from build123d import *

# Parameters (mm, degrees)
SKETCH051_W         = 21.9
SKETCH051_H         = 24
PAD014_DEPTH        = 4
SKETCH052_R         = 5.9
POCKET015_DEPTH     = 1.2
SKETCH053_W         = 16
SKETCH053_H         = 6
SKETCH053_W_2       = 4
POCKET016_DEPTH     = 1.2
HOLE022_D           = 2.8
HOLE022_DEPTH       = 25
HOLE022_CBORE_D     = 6
HOLE022_CBORE_DEPTH = 2
FILLET027_R         = 2


with BuildPart() as part:
    # Sketch051 → Pad014 (new body)
    with BuildSketch(Plane.XY):
        with Locations((11.05, 0)):
            Rectangle(SKETCH051_W, SKETCH051_H)
    extrude(amount=PAD014_DEPTH)

    # Sketch052 (on Face6 of Pad014) → Pocket015 (cut)
    with BuildSketch(Plane.XY.offset(4)):
        with Locations((7.5, 0)):
            Circle(SKETCH052_R)
    pocket015 = extrude(amount=-POCKET015_DEPTH, mode=Mode.SUBTRACT)

    # Mirrored025: Pocket015 across Sketch052 V_Axis
    add(pocket015.mirror(Plane(origin=(0, 0, 4), x_dir=(0, 0, 1), z_dir=(1, 0, 0))), mode=Mode.SUBTRACT)

    # Sketch053 (on Face5 of Mirrored025) → Pocket016 (cut)
    with BuildSketch(Plane.XY.offset(4)):
        with Locations((0, 3)):
            Rectangle(SKETCH053_W, SKETCH053_H)
        with Locations((0, 9)):
            Rectangle(SKETCH053_W_2, SKETCH053_H)
    extrude(amount=-POCKET016_DEPTH, mode=Mode.SUBTRACT)

    # Hole022
    with Locations(Plane(origin=(0, 0, 0), x_dir=(1, 0, 0), z_dir=(0, 0, -1))):
        with Locations((16.2, 8.2), (16.2, -8.2), (3.8, 8.2), (3.8, -8.2)):
            hole022 = CounterBoreHole(HOLE022_D / 2, HOLE022_CBORE_D / 2, HOLE022_CBORE_DEPTH, depth=HOLE022_DEPTH)

    # Mirrored026: Hole022 across Sketch054 V_Axis
    add(hole022.mirror(Plane(origin=(0, 0, 0), x_dir=(0, 0, -1), z_dir=(1, 0, 0))), mode=Mode.SUBTRACT)

    # Fillet027
    fillet027_edges = [part.edges().sort_by_distance(p)[0] for p in [
        (22, 12, 2),
        (22, -12, 2),
    ]]
    fillet(fillet027_edges, radius=FILLET027_R)


solid = part.part
Geometry check sheet. Reference: the model listing, model coordinates, mm. A direction names the side the tool comes from. Round coordinates to 2 decimals unless told otherwise and drop trailing zeros. Loops run counter-clockwise (first coordinate to the right, second up) from the corner with the lowest first, then second, coordinate; pieces in that order, holes last. Notation, with made-up numbers: (-5, 4.25) -> (8, 4.25) arc R28 ccw to (8, 23.25) -> close; hole circle Ø8 at (72, 1). An arc over 180 degrees is marked (long way). Answer as a JSON object with one key per item and string values. Group by question number.
Item 1: Set-up check for faces 1 (the face through (4, -10, 2)), 2 (the face through (1, 0, 3)), 3 (the face through (11.35, -4.47, 3.41)), 4 (the face through (22, 0, 2)): record each of +Z, -Z, +X, -X, +Y, -Y from which the full face is reachable in a straight line by a thin tool's end or side.
Item 2: Cross-section at C-C, the plane z = 0.8. Record the cut outline in (x, y).
Item 3: Release check for a two-part mould opening along Y. For faces 5 (the face through (15, -7, 2)), 6 (the face through (2, 9, 3)), 7 (the face through (21.4, 11.43, 2.03)) record: pulls with the +Y half, pulls with the -Y half, needs draft (parallel to the pull), parting line crosses it, or undercut.
Item 4: Thickness scan on line 1 along Y through (x, z) = (16.2, 2.9); line 2 along X through (y, z) = (8.2, 3.55); line 3 along X through (y, z) = (-8.2, 2.8). Record the ranges inside material, lowest first.
Item 5: Cross-section at A-A, the plane y = -8.2. Record the cut outline in (x, z), plus the area to 3 significant figures.
Item 6: Depth check by flat-ended pin: pin 1 Ø3 at (x, y) = (3.8, 8.2) entering from +Z; pin 2 Ø2 at (x, y) = (3.8, -8.2) entering from -Z; pin 3 Ø5.5 at (x, y) = (3.8, -8.2) entering from -Z; pin 4 Ø4 at (x, y) = (4.5, 3) entering from +Z. Enter the tip coordinate at first touch or a pass-through.
Item 7: Cross-section at B-B, the plane x = 16.2. Record the cut outline in (y, z).
Item 8: Cross-section at D-D, the plane x = 7.5. Record the cut outline in (y, z), plus the area to 3 significant figures.
Determined:
{
 "1": {"face 1": "-Z", "face 2": "+Z, -X, +Y", "face 3": "+Z", "face 4": "+Z, -Z, +X, +Y, -Y"},
 "2": {"outline": "(0.1, -12) -> (20, -12) arc R2 ccw to (22, -10) -> (22, 10) arc R2 ccw to (20, 12) -> (0.1, 12) -> close; hole circle Ø6 at (3.8, -8.2); hole circle Ø6 at (3.8, 8.2); hole circle Ø6 at (16.2, -8.2); hole circle Ø6 at (16.2, 8.2)"},
 "3": {"face 5": "undercut", "face 6": "needs draft", "face 7": "pulls with the +Y half"},
 "4": {"line 1": "y = -12 to -9.6, -6.8 to 6.8, 9.6 to 12", "line 2": "x = 2 to 2.4, 5.2 to 14.8, 17.6 to 22", "line 3": "x = 0.1 to 2.4, 5.2 to 14.8, 17.6 to 22"},
 "5": {"outline": "(0.1, 0) -> (0.8, 0) -> (0.8, 2) -> (2.4, 2) -> (2.4, 4) -> (0.1, 4) -> close; (5.2, 2) -> (6.8, 2) -> (6.8, 0) -> (13.2, 0) -> (13.2, 2) -> (14.8, 2) -> (14.8, 4) -> (5.2, 4) -> close; (17.6, 2) -> (19.2, 2) -> (19.2, 0) -> (22, 0) -> (22, 4) -> (17.6, 4) -> close", "area": "52.4 mm²"},
 "6": {"pin 1": "stops at z = 4", "pin 2": "passes through", "pin 3": "stops at z = 2", "pin 4": "stops at z = 2.8"},
 "7": {"outline": "(-12, 0) -> (-11.2, 0) -> (-11.2, 2) -> (-9.6, 2) -> (-9.6, 4) -> (-12, 4) -> close; (-6.8, 2) -> (-5.2, 2) -> (-5.2, 0) -> (5.2, 0) -> (5.2, 2) -> (6.8, 2) -> (6.8, 4) -> (-6.8, 4) -> close; (9.6, 2) -> (11.2, 2) -> (11.2, 0) -> (12, 0) -> (12, 4) -> (9.6, 4) -> close"},
 "8": {"outline": "(-12, 0) -> (12, 0) -> (12, 4) -> (6, 4) -> (6, 2.8) -> (-5.9, 2.8) -> (-5.9, 4) -> (-12, 4) -> close", "area": "81.7 mm²"}
}
